Model file for the job. Use its own axes, mm. Give positions to 0.01 mm unless a question says otherwise; leave off trailing zeros. Order: outer loops, then holes, each group sorted by start corner. A loop starts at its lowest first (then second) coordinate and runs counter-clockwise, first axis right, second up. Notation, with made-up numbers: M 41,22 L 71,22 A12 ccw 71,34 Z; hole C 30,4.5 d2. An arc over 180 degrees is marked long. Return JSON: item names as keys, results as strings. Group by question number.
1. Slice it at B-B on y = 1.95. Give the number of separate pieces and of enclosed holes in the cut face, then the cut area to 3 significant figures.
2. Pin check, flat tips, straight feed: pin 1 (11.5 mm diameter, centred on x = -36.54, z = 0, fed in from +Y); pin 2 (23.5 mm diameter, centred on x = -19.5, z = 14, fed in from -Y); pin 3 (3 mm diameter, centred on x = -5, y = 1.5, fed in from +Z). Stop position of each tip, or through.
3. Slice it at A-A on z = 0. List the corners of the cut face in (x, y).
4. Wall check: probe 1 along X at (y, z) = (0.95, 22); probe 2 along Z at (x, y) = (-14, 1.45); probe 3 along Z at (x, y) = (-45, 0.95). Give the ranges that are in metal, low to high. Write a range as [from, to].
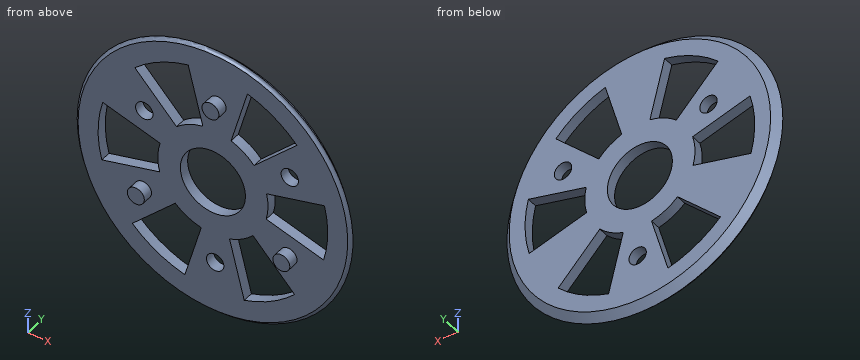
from build123d import *

# Parameters (mm, degrees)
SKETCH2_R           = 9.5
BOSS_EXTRUDE1_DEPTH = 3
SKETCH3_R           = 2.4765
BOSS_EXTRUDE2_DEPTH = 6
SKETCH5_R           = 2.54
CUT_EXTRUDE1_DEPTH  = 3


with BuildPart() as part:
    # Sketch1 → Revolve1 (revolve)
    with BuildSketch(Plane.XY, mode=Mode.PRIVATE) as revolve1_sk:
        with BuildLine():
            Line((-3, 3), (-3, 0))
            Line((-3, 0), (2.833330973, 0))
            ThreePointArc((2.833330973, 0), (3.099026965, 0.641446866), (3.74047383, 0.907142857))
            Line((3.74047383, 0.907142857), (1.647616688, 3))
            Line((1.647616688, 3), (-3, 3))
        make_face()
    revolve(revolve1_sk.sketch.rotate(Axis((-36.536669027, 18.916479231, 0), (0, -1, 0)), 180), axis=Axis((-36.536669027, 18.916479231, 0), (0, -1, 0)))

    # Sketch2 → Boss-Extrude1 (add)
    with BuildSketch(Plane(origin=(0, 0, 0), x_dir=(1, 0, 0), z_dir=(0, 1, 0))):
        with BuildLine():
            Line((-20.867712208, -3.717876844), (-3.835179752, -7.99934189))
            ThreePointArc((-3.835179752, -7.99934189), (-6.912459925, -15.993220643), (-11.907531207, -22.951741583))
            Line((-11.907531207, -22.951741583), (-24.531535953, -10.733852798))
            ThreePointArc((-24.531535953, -10.733852798), (-27.594601894, -13.393216618), (-31.225026168, -15.202804549))
            Line((-31.225026168, -15.202804549), (-26.411510933, -32.106978136))
            ThreePointArc((-26.411510933, -32.106978136), (-35.048905375, -33.632773165), (-43.787287916, -32.875604894))
            Line((-43.787287916, -32.875604894), (-39.473539012, -15.833938572))
            ThreePointArc((-39.473539012, -15.833938572), (-43.573178883, -14.485383842), (-47.167458429, -12.096492578))
            Line((-47.167458429, -12.096492578), (-59.432790875, -24.680852412))
            ThreePointArc((-59.432790875, -24.680852412), (-65.164474953, -17.715123462), (-68.840755241, -9.47749362))
            Line((-68.840755241, -9.47749362), (-51.939863017, -4.698981901))
            ThreePointArc((-51.939863017, -4.698981901), (-52.638650424, -0.254972715), (-52.080918658, 4.208933284))
            Line((-52.080918658, 4.208933284), (-69.114911822, 8.487341623))
            ThreePointArc((-69.114911822, 8.487341623), (-65.689685641, 16.836819584), (-60.169485242, 23.976381487))
            Line((-60.169485242, 23.976381487), (-47.536935944, 11.761502615))
            ThreePointArc((-47.536935944, 11.761502615), (-44.010986284, 14.264410171), (-39.946180469, 15.738934136))
            Line((-39.946180469, 15.738934136), (-44.764676694, 32.64470495))
            ThreePointArc((-44.764676694, 32.64470495), (-36.044934422, 33.662071661), (-27.358629805, 32.390437902))
            Line((-27.358629805, 32.390437902), (-31.667700916, 15.350308321))
            ThreePointArc((-31.667700916, 15.350308321), (-27.981833761, 13.643812135), (-24.840179389, 11.069369727))
            Line((-24.840179389, 11.069369727), (-12.58348556, 23.656328398))
            ThreePointArc((-12.58348556, 23.656328398), (-7.387085692, 16.842762923), (-4.079178242, 8.938017868))
            Line((-4.079178242, 8.938017868), (-20.977889223, 4.154899158))
            ThreePointArc((-20.977889223, 4.154899158), (-20.434245789, 0.225348329), (-20.867712208, -3.717876844))
        make_face()
        with Locations(Location((-36.536669027, 0, 0), (0, 0, 180))):
            Circle(SKETCH2_R, mode=Mode.SUBTRACT)
    extrude(amount=BOSS_EXTRUDE1_DEPTH)

    # Sketch3 → Boss-Extrude2 (add)
    with BuildSketch(Plane(origin=(0, 3, 0), x_dir=(1, 0, 0), z_dir=(0, 1, 0))):
        with Locations(Location((-35.151038514, -24.531821511, 0), (0, 0, 180))):
            Circle(SKETCH3_R)
        with Locations(Location((-56.941625658, 11.951020157, 0), (0, 0, 180))):
            Circle(SKETCH3_R)
        with Locations(Location((-14.451264399, 12.580801354, 0), (0, 0, 180))):
            Circle(SKETCH3_R)
    extrude(amount=-BOSS_EXTRUDE2_DEPTH)

    # Sketch5 → Cut-Extrude1 (cut)
    with BuildSketch(Plane(origin=(0, 3, 0), x_dir=(1, 0, 0), z_dir=(0, 1, 0))):
        with Locations(Location((-35.8782472, 24.531821511, 0), (0, 0, 180))):
            Circle(SKETCH5_R)
        with Locations(Location((-14.087660056, -11.951020157, 0), (0, 0, 180))):
            Circle(SKETCH5_R)
        with Locations(Location((-56.578021315, -12.580801354, 0), (0, 0, 180))):
            Circle(SKETCH5_R)
    extrude(amount=-CUT_EXTRUDE1_DEPTH, mode=Mode.SUBTRACT)


solid = part.part
Result:
{
 "1": {"separate pieces": "1", "enclosed holes": "10", "area": "3,130 mm2"},
 "2": {"pin 1": "passes through", "pin 2": "stops at y = 0", "pin 3": "stops at z = 26.7"},
 "3": {"outline": "M -76.81,0.91 A0.91 cw -75.91,0 L -70.07,0 L -70.07,3 L -74.72,3 Z; M -52.64,0 L -46.04,0 L -46.04,3 L -52.64,3 Z; M -27.04,0 L -20.43,0 L -20.43,3 L -27.04,3 Z; M -3,0 L 2.83,0 A0.91 cw 3.74,0.91 L 1.65,3 L -3,3 Z"},
 "4": {"probe 1": "x = [-70.22, -56.82], [-41.03, -29.29], [-12.89, -2.85]", "probe 2": "z = [-32.72, -24.84], [-22.2, -6.13], [5.44, 9.41], [14.49, 20.93], [24.84, 32.72]", "probe 3": "z = [-39.33, -32.45], [-13.7, -4.32], [4.32, 13.7], [32.45, 39.33]"}
}
